from build123d import *

# Parameters (mm, degrees)
F0_W     = 508
F0_H     = 508
F1_DEPTH = 25.4
F2_W     = 76.2
F2_H     = 76.2
F3_DEPTH = 762
F4_R     = 254
F5_DEPTH = 12.7
F6_R     = 6.35
F7_DEPTH = 152.4


with BuildPart() as f1:
    # F0 (on Top) → F1 (new body)
    with BuildSketch(Plane.XY):
        Rectangle(F0_W, F0_H)
    extrude(amount=F1_DEPTH)

    # F2 (on face) → F3 (join)
    with BuildSketch(Plane.XY.offset(25.4)):
        Rectangle(F2_W, F2_H)
    extrude(amount=F3_DEPTH)

    # F4 (on face) → F5 (join)
    with BuildSketch(Plane.XY.offset(787.4)):
        Circle(F4_R)
    extrude(amount=F5_DEPTH)

    # F6 (on face) → F7 (cut)
    with BuildSketch(Plane.XY.offset(800.1)):
        Circle(F6_R)
    extrude(amount=-F7_DEPTH, mode=Mode.SUBTRACT)


solid = f1.part
Build history of the part. All positions in model axes, mm. A direction names the side the tool comes from. Round coordinates to 2 decimals unless told otherwise and drop trailing zeros. Order: outer loops, then holes, each group sorted by start corner. A loop starts at its lowest first (then second) coordinate and runs counter-clockwise, first axis right, second up. Notation, with made-up numbers: M 7.25,55.25 L 42.25,55.25 A10 cw 42.25,68.25 Z; hole C 2,14.5 d3. An arc over 180 degrees is marked long. Use CSV: the item, a comma, the result in double quotes. Start each with the question number.
(1) Flat gauge pins, fed straight in: P1, Ø1.5, axis at y = 11, z = 687.5, coming from the -X side; P2, Ø7.5, axis at x = 0, y = 0, coming from the +Z side; P3, Ø1.5, axis at y = -39, z = 379, coming from the -X side. Where does each tip first touch, or does it go through?
(2) Mould opens along Z. For faces 1 (the face through (-4, 254, 13)), 2 (the face through (-1, -38.1, 401)), 3 (the face through (53, 4, 25.4)), 4 (the face through (-4, 4, 0)) say: +Z half, -Z half, draft (parallel to the pull), parting line (faces both ways), or undercut.
(3) Cut at A-A on x = -101.5. List the corners of the cut face in (y, z).
(4) Cut at B-B on y = 55.5. List the corners of the cut face in (x, z).
(5) Cut at C-C on z = 751.5. List the corners of the cut face in (x, y).
(6) Cut at D-D on z = 63.5. List the corners of the cut face in (x, y).
(7) Drill centre lines: probe 1 along Z at (x, y) = (190.5, 149); probe 2 along Y at (x, z) = (0, 731); probe 3 along Z at (x, y) = (-136.5, -228.5). Where is each one in solid material? Low to high.
(8) Tool access for faces 5 (the face through (38.1, -1, 401)), 6 (the face through (53, 4, 800.1)), 7 (the face through (-38.1, -1, 401)), 8 (the face through (-1, 38.1, 401)), 9 (the face through (-55.06, -247.96, 793.66)): list every direction of +Z, -Z, +X, -X, +Y, -Y with a clear straight run to the whole face (end or side of a thin tool).
Findings:
1,P1,"stops at x = -38.1"
1,P2,"stops at z = 647.7"
1,P3,"passes through"
2,face 1,"draft"
2,face 2,"undercut"
2,face 3,"undercut"
2,face 4,"-Z half"
3,outline,"M -254,0 L 254,0 L 254,25.4 L -254,25.4 Z; M -232.84,787.4 L 232.84,787.4 L 232.84,800.1 L -232.84,800.1 Z"
4,outline,"M -254,0 L 254,0 L 254,25.4 L -254,25.4 Z; M -247.86,787.4 L 247.86,787.4 L 247.86,800.1 L -247.86,800.1 Z"
5,outline,"M -38.1,-38.1 L 38.1,-38.1 L 38.1,38.1 L -38.1,38.1 Z; hole C 0,0 d12.7"
6,outline,"M -38.1,-38.1 L 38.1,-38.1 L 38.1,38.1 L -38.1,38.1 Z"
7,probe 1,"z = 0 to 25.4, 787.4 to 800.1"
7,probe 2,"y = -38.1 to -6.35, 6.35 to 38.1"
7,probe 3,"z = 0 to 25.4"
8,face 5,"+X, +Y, -Y"
8,face 6,"+Z, +X, -X, +Y, -Y"
8,face 7,"-X, +Y, -Y"
8,face 8,"+X, -X, +Y"
8,face 9,"+Z"
